```python
from build123d import *

# Parameters (mm, degrees)
SKETCH_1_R          = 15
EXTRUDE_1_DEPTH     = 10
SKETCH_2_R          = 1.95
EXTRUDE_2_DEPTH     = 4
SKETCH_3_W          = 3.1
SKETCH_3_H          = 25.258877381
CUT_EXTRUDE_1_DEPTH = 8


with BuildPart() as part:
    # Sketch 1 → Extrude 1 (new body)
    with BuildSketch(Plane.XY):
        Circle(SKETCH_1_R)
    extrude(amount=EXTRUDE_1_DEPTH)

    # Sketch 2 → Extrude 2 (add)
    with BuildSketch(Plane(origin=(0, 0, 0), x_dir=(-1, 0, 0), z_dir=(0, 0, -1))):
        with Locations(Location((0, 0, 0), (0, 0, 180))):
            Circle(SKETCH_2_R)
    extrude(amount=EXTRUDE_2_DEPTH)

    # Sketch 3 → Cut-Extrude 1 (cut)
    with BuildSketch(Plane.XY.offset(10)):
        Polygon((29.256878851, 7.876369741), (5.234258923, 0.070947372), (4.27630624, 3.019222572), (28.298926168, 10.824644942), align=None)
        with Locations((0, 17.629438691)):
            Rectangle(SKETCH_3_W, SKETCH_3_H)
        Polygon((16.531745534, -25.391013173), (1.68494992, -4.956152113), (4.192902603, -3.134017831), (19.039698217, -23.568878891), align=None)
        Polygon((-19.039698217, -23.568878891), (-4.192902603, -3.134017831), (-1.68494992, -4.956152113), (-16.531745534, -25.391013173), align=None)
        Polygon((-28.298926168, 10.824644942), (-4.27630624, 3.019222572), (-5.234258923, 0.070947372), (-29.256878851, 7.876369741), align=None)
    extrude(amount=-CUT_EXTRUDE_1_DEPTH, mode=Mode.SUBTRACT)


solid = part.part
```
Read the model definition and answer for the solid it produces. Units are mm, in the model's axes. A direction names the side the tool comes from. Round coordinates to 2 decimals unless told otherwise and drop trailing zeros. Write each loop counter-clockwise with the first axis right and the second up, starting at its lowest first coordinate (ties: lowest second). Pieces come first, ordered by that corner, then holes. Notation, with made-up numbers: M -19.5,3 L -0.5,3 A32 ccw -0.5,42 Z; hole C 50,70 d9. An arc over 180 degrees is marked long. One line per item, written item: value.
Q1. Find section C-C on y = -7.75. Write down the section's boundary in (x, z), plus the area to 3 significant figures.
Data:
outline: M -12.84,0 L 12.84,0 L 12.84,10 L 7.55,10 L 7.55,2 L 3.71,2 L 3.71,10 L -3.71,10 L -3.71,2 L -7.55,2 L -7.55,10 L -12.84,10 Z
area: 196 mm2
Q2. Flat-ended cylindrical pins translate along their axes: pin 1 Ø6.5 at (x, y) = (-10.5, 3.5) entering from +Z; pin 2 Ø3 at (y, z) = (-4, 4) entering from -X; pin 3 Ø4 at (y, z) = (10, 8) entering from +X; pin 4 Ø6 at (y, z) = (-10, 5) entering from +X. Find the tip coordinate at first contact, or state that the pin passes through.
Data:
pin 1: z = 10
pin 2: x = -14.79
pin 3: x = 12.69
pin 4: x = 13.27
Q3. Straight lines are drawn through the part: line 1 (X direction, y = -9, z = 7.5); line 2 (Z direction, x = 7, y = 2.25); line 3 (Z direction, x = -11, y = 9.5). For each, find the intervals that lie inside material, in ascending order. Write a range as [from, to].
Data:
line 1: [-12, -8.45], [-4.62, 4.62], [8.45, 12]
line 2: [0, 2]
line 3: [0, 10]
Q4. Find section B-B on x = 0. Write down the section's boundary in (y, z).
Data:
outline: M -15,0 L -1.95,0 L -1.95,-4 L 1.95,-4 L 1.95,0 L 15,0 L 15,2 L 5,2 L 5,10 L -15,10 Z
Q5. Find section D-D on x = -3.5. Write down the section's boundary in (y, z), plus the area to 3 significant figures.
Data:
outline: M -14.59,0 L 14.59,0 L 14.59,10 L -3.64,10 L -3.64,2 L -7.45,2 L -7.45,10 L -14.59,10 Z
area: 261 mm2
Q6. For a pull along X with two mould halves and no side action, classify faces 4 (the flat face through (3, 0, 0)), 5 (the cylindrical face through (-1.437, -1.318, -1.972)), 6 (the flat face through (3, -4, 6)) as +X half, -X half, draft (parallel to the pull), parting line (faces both ways), or undercut.
Data:
face 4: draft
face 5: parting line
face 6: undercut
Q7. Find section A-A on z = 5.5. Write down the section's boundary in (x, y), plus the area to 3 significant figures.
Data:
outline: M -14.67,3.14 A15 ccw -10.02,-11.16 L -4.19,-3.13 L -1.68,-4.96 L -7.52,-12.98 A15 ccw 7.52,-12.98 L 1.68,-4.96 L 4.19,-3.13 L 10.02,-11.16 A15 ccw 14.67,3.14 L 5.23,0.07 L 4.28,3.02 L 13.71,6.08 A15 ccw 1.55,14.92 L 1.55,5 L -1.55,5 L -1.55,14.92 A15 ccw -13.71,6.08 L -4.28,3.02 L -5.23,0.07 Z
area: 552 mm2
Q8. Which of the six approach directions +Z, -Z, +X, -X, +Y, -Y give full straight-line access (tool end or side, diameter ignored) to faces 1 (the flat face through (-3, -4, 6)), 2 (the flat face through (0, 5, 6)), 3 (the flat face through (0, 0, 10))?
Data:
face 1: +Z
face 2: +Z, +Y
face 3: +Z, +X, -X, +Y, -Y
